from build123d import *

# Parameters (mm, degrees)
F0_W     = 66.933575
F0_H     = 21.369922
F1_DEPTH = 50.8
F3_DEPTH = 76.2
F4_W     = 37.397362
F4_H     = 20.0979
F5_DEPTH = 101.6
F6_W     = 47.573516
F6_H     = 30.274053
F7_DEPTH = 10.16


with BuildPart() as f1:
    # F0 (on Front) → F1 (new body)
    with BuildSketch(Plane.XZ):
        with Locations((-1.971668, 8.522528)):
            Rectangle(F0_W, F0_H)
    extrude(amount=-F1_DEPTH)

    # F2 (on face) → F3 (cut)
    with BuildSketch(Plane(origin=(-35.438456, 0, 0), x_dir=(0, -1, 0), z_dir=(-1, 0, 0))):
        Polygon((0, 19.207489), (-50.8, 19.207489), (0, 8.522528), align=None)
    extrude(amount=-F3_DEPTH, mode=Mode.SUBTRACT)

    # F4 (on face) → F5 (join)
    with BuildSketch(Plane(origin=(0, 0, -2.162433), x_dir=(1, 0, 0), z_dir=(0, 0, -1))):
        with Locations((-3.30725, -25.185978)):
            Rectangle(F4_W, F4_H)
    extrude(amount=F5_DEPTH)

    # F6 (on face) → F7 (join)
    with BuildSketch(Plane(origin=(0, 0, -103.762433), x_dir=(1, 0, 0), z_dir=(0, 0, -1))):
        with Locations((-3.561654, -24.422762)):
            Rectangle(F6_W, F6_H)
    extrude(amount=F7_DEPTH)


solid = f1.part
Design review of the part built by this model. Coordinates are the model's own, in mm. A direction names the side the tool comes from. Round coordinates to 2 decimals unless told otherwise and drop trailing zeros. Write each loop counter-clockwise with the first axis right and the second up, starting at its lowest first coordinate (ties: lowest second). Pieces come first, ordered by that corner, then holes. Notation, with made-up numbers: (5.5, -34) - (59.5, -34) arc R32 cw to (59.5, -8) - close; hole circle Ø3 at (50.25, 26.5). An arc over 180 degrees is marked (long way). Use a Markdown table: item, result. Add a question column.
1. Clearance check with flat-ended pins moving along their axes: pin 1 (3 mm diameter, centred on x = -1.5, z = -109, fed in from +Y); pin 2 (8 mm diameter, centred on x = 4.5, z = -108.5, fed in from -Y); pin 3 (6 mm diameter, centred on y = 30, z = -77, fed in from -X). State where each tip first meets the part, or that it passes through.
2. For faces 1 (the face through (20.225, 25, -109)), 2 (the face through (-4, 39.56, -109)), 3 (the face through (-22.006, 25, -52)), list the 3-axis set-ups (+Z, -Z, +X, -X, +Y, -Y) from which the entire face can be reached by the end or side of a thin tool; tool diameter is ignored.
3. We need section A-A (x = 17.5). State the section outline as (y, z) points.
4. We need section D-D (y = 22.5). State the section outline as (x, z) points, then the cut area to 3 significant figures.
5. Wall thickness on probe 1 along Y at (x, z) = (11, -49); probe 2 along X at (y, z) = (22, -106); probe 3 along Y at (x, z) = (-27, -107.5): over which ranges is each line inside the solid? List them lowest first.
6. We need section B-B (y = 11.5). State the section outline as (x, z) points.
7. Mouldability with a two-part tool opening along Z and no side actions: class faces 4 (the face through (15.391, 25, -52)), 5 (the face through (-4, 9.286, -109)), 6 (the face through (-4, 24, -113.922)) as +Z half, -Z half, draft (parallel to the pull), parting line (faces both ways), or undercut.
8. We need section C-C (x = -5). State the section outline as (y, z) points.
Output:
| question | item | result |
|---|---|---|
| 1 | pin 1 | stops at y = 39.56 |
| 1 | pin 2 | stops at y = 9.29 |
| 1 | pin 3 | stops at x = -22.01 |
| 2 | face 1 | -Z, +X, +Y, -Y |
| 2 | face 2 | -Z, +X, -X, +Y |
| 2 | face 3 | -X, +Y, -Y |
| 3 | outline | (0, -2.16) - (50.8, -2.16) - (50.8, 19.21) - (0, 8.52) - close; (9.29, -113.92) - (39.56, -113.92) - (39.56, -103.76) - (9.29, -103.76) - close |
| 4 | outline | (-35.44, -2.16) - (-22.01, -2.16) - (-22.01, -103.76) - (-27.35, -103.76) - (-27.35, -113.92) - (20.23, -113.92) - (20.23, -103.76) - (15.39, -103.76) - (15.39, -2.16) - (31.5, -2.16) - (31.5, 13.26) - (-35.44, 13.26) - close |
| 4 | area | 5,310 mm2 |
| 5 | probe 1 | y = 15.14 to 35.23 |
| 5 | probe 2 | x = -27.35 to 20.23 |
| 5 | probe 3 | y = 9.29 to 39.56 |
| 6 | outline | (-35.44, -2.16) - (31.5, -2.16) - (31.5, 10.94) - (-35.44, 10.94) - close; (-27.35, -113.92) - (20.23, -113.92) - (20.23, -103.76) - (-27.35, -103.76) - close |
| 7 | face 4 | undercut |
| 7 | face 5 | draft |
| 7 | face 6 | -Z half |
| 8 | outline | (0, -2.16) - (15.14, -2.16) - (15.14, -103.76) - (9.29, -103.76) - (9.29, -113.92) - (39.56, -113.92) - (39.56, -103.76) - (35.23, -103.76) - (35.23, -2.16) - (50.8, -2.16) - (50.8, 19.21) - (0, 8.52) - close |
